The listing builds one solid part. Answer for the finished solid, in the listing's coordinates (mm). Round coordinates to 2 decimals unless told otherwise and drop trailing zeros. Loops run counter-clockwise (first coordinate to the right, second up) from the corner with the lowest first, then second, coordinate; pieces in that order, holes last. Notation, with made-up numbers: M -26,-34.5 L -16,-34.5 A21 cw -16,-25.5 Z; hole C -25,22 d4. An arc over 180 degrees is marked long. Answer as a JSON object with one key per item and string values.
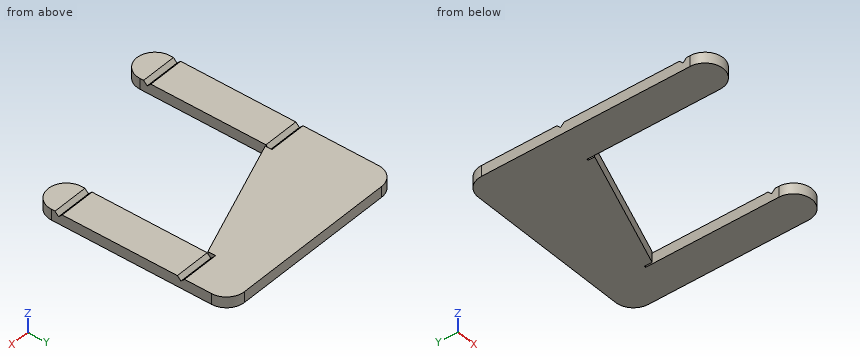
Autodesk Fusion 360 part; units mm, degrees
sketch "Sketch1" plane through (0, 0, 0) normal (0, 0, 1) x (1, 0, 0)
  line L0 (56, 13.5) -> (56, 28)
  line L1 (56, 28) -> (0, 28)
  line L2 (0, 28) -> (0, 0)
  line L3 (0, 0) -> (10, 0)
  line L4 (10, 0) -> (46, 0) construction
  line L5 (0, 0) -> (0, -35)
  arc A0 (0, -35) -> (10, -35) centre (5, -35) ccw
  line L6 (10, -35) -> (10, 0)
  line L7 (46, 0) -> (46, 13.5) construction
  line L8 (46, 13.5) -> (56, 13.5)
  line L9 (46, 13.5) -> (10, 0)
  line L10 (46, 13.5) -> (46, -21.5)
  arc A1 (46, -21.5) -> (56, -21.5) centre (51, -21.5) ccw
  line L11 (56, -21.5) -> (56, 13.5)
  line L12 (0, -33) -> (10, -33) construction
  line L13 (46, -19.5) -> (56, -19.5) construction
  line L14 (46, 15.5) -> (56, 15.5)
  line L15 (0, 2) -> (10, 2)
  line L16 (0, -32) -> (10, -32)
  line L17 (0, -34) -> (10, -34)
  line L18 (46, -18.5) -> (56, -18.5)
  line L19 (46, -20.5) -> (56, -20.5)
  line L20 (46, 15.5) -> (46, 13.5)
  line L21 (46, 15.5) -> (45.6, 15.5)
  line L22 (45.6, 15.5) -> (45.6, 13.35)
  line L23 (10, 0) -> (10, 2)
  line L24 (10, 2) -> (10.4, 2)
  line L25 (10.4, 2) -> (10.4, 0.15)
  dimension "d1" = 28
  dimension "d5" = 10
  dimension "d6" = 10
  dimension "d7" = 36
  dimension "d8" = 13.5
  dimension "d11" = 33
  dimension "d12" = 2
  dimension "d13" = 2
  dimension "d14" = 33
  dimension "d20" = 2
  dimension "d21" = 2
  dimension "d27" = 2
  dimension "d28" = 0.4
  dimension "d29" = 2
  dimension "d30" = 0.4
extrude "Extrude1" add sketch "Sketch1" against normal blind 3 contours L0 L8 L14 L20 | L8 L10 L11 L18 | L0 L1 L2 L9 L14 L15 L21 L22 L24 L25 | L10 L11 L18 L19 | L10 A1 L11 L19 | L2 L3 L15 L23 | L3 L5 L6 L16 | L5 L6 L16 L17 | L5 A0 L6 L17
extrude "Extrude2" cut sketch "Sketch1" against normal blind 1 contours L0 L8 L14 L20 | L10 L11 L18 L19 | L2 L3 L15 L23 | L5 L6 L16 L17
chamfer "Chamfer1" distance 1 angle 45 8 edges at (5, -32, -1) (5, -34, -1) (5, 2, -1) (5, 0, -1) (51, 13.5, -1) (51, 15.5, -1) (51, -20.5, -1) (51, -18.5, -1)
fillet "Fillet1" radius 5 2 edges at (56, 28, -1.5) (0, 28, -1.5)
equation "d13 = d12"
equation "d14 = d11"
Item 1: The part is cut by section C-C (y = -23). Give the vertices of the cut face in (x, z).
Values follow:
{"outline": "M 0,-3 L 10,-3 L 10,0 L 0,0 Z; M 46.23,-3 L 55.77,-3 L 55.77,0 L 46.23,0 Z"}
Item 2: The part is cut by section B-B (x = 40). Give the vertices of the cut face in (y, z), then the cut area to 4 significant figures.
Values follow:
{"outline": "M 11.25,-3 L 28,-3 L 28,0 L 11.25,0 Z", "area": "50.25 mm^2"}
Item 3: The part is cut by section A-A (y = 3.5). Give the vertices of the cut face in (x, z).
Values follow:
{"outline": "M 0,-3 L 19.33,-3 L 19.33,0 L 0,0 Z; M 46,-3 L 56,-3 L 56,0 L 46,0 Z"}
Item 4: Straight lines are drawn through the part: line 1 (X direction, y = 15, z = -2.15); line 2 (X direction, y = -11, z = -0.8); line 3 (Y direction, x = 9.5, z = -0.15). For each, find the intervals that lie inside material, in ascending order.
Values follow:
{"line 1": "0 to 45.6, 46 to 56", "line 2": "0 to 10, 46 to 56", "line 3": "-37.18 to -33.85, -32.15 to 0.15, 1.85 to 28"}
Item 5: The part is cut by section D-D (x = 12). Give the vertices of the cut face in (y, z).
Values follow:
{"outline": "M 0.75,-3 L 28,-3 L 28,0 L 0.75,0 Z"}
Item 6: A flat-ended cylindrical pin translates along its axis: P1, Ø1.5, axis at x = 48, z = -2, coming from the -Y side. Find the tip coordinate at first contact, or state that the pin passes through.
Values follow:
{"P1": "y = -25.97"}
